Geometry check sheet. Reference: the model listing, model coordinates, mm. Face numbers are marked on the shaded views. A direction names the side the tool comes from. Give positions to 0.01 mm unless a question says otherwise; leave off trailing zeros. Loops run counter-clockwise (first coordinate to the right, second up) from the corner with the lowest first, then second, coordinate; pieces in that order, holes last. Notation, with made-up numbers: (87.5, 85.5) - (107.5, 85.5) arc R20 cw to (107.5, 122.5) - close; hole circle Ø4 at (59.25, 72.25). An arc over 180 degrees is marked (long way). One line per question, with ' | ' between items. Start each with the question number.
from build123d import *

# Parameters (mm, degrees)
F0_R     = 5
F1_DEPTH = 5
F2_W     = 3
F2_H     = 1.5
F3_DEPTH = 3
F4_R     = 0.5
F5_DEPTH = 25


with BuildPart() as f1:
    # F0 (on Top) → F1 (new body)
    with BuildSketch(Plane.XY):
        Circle(F0_R)
    extrude(amount=F1_DEPTH)

    # F2 (on face) → F3 (join)
    with BuildSketch(Plane.XY.offset(5)):
        with Locations((0, -2.75)):
            Rectangle(F2_W, F2_H)
    extrude(amount=F3_DEPTH)

    # F4 (on face) → F5 (cut)
    with BuildSketch(Plane.XY.offset(5)):
        Circle(F4_R)
    extrude(amount=-F5_DEPTH, mode=Mode.SUBTRACT)


solid = f1.part
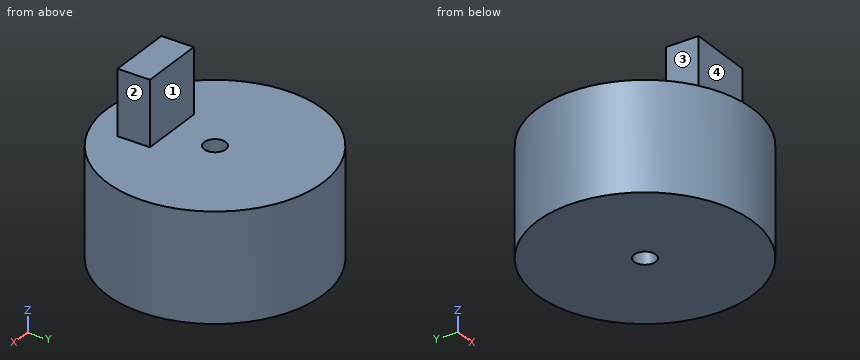
(1) Section check B-B, the plane z = 1. Record the boundary of the cut face in (x, y), and give its area (3 significant figures).
(2) Section check D-D, the plane x = 4. Record the boundary of the cut face in (y, z), and give its area (3 significant figures).
(3) Tool access check on the marked faces 1, 2, 3 and 4. Record the directions out of +Z, -Z, +X, -X, +Y, -Y that give a thin tool (end or side, any length) a straight path to the whole face; none if there is none.
(4) Depth check by flat-ended pin: pin 1 Ø1.6 at (y, z) = (-2.5, 6.5) entering from +X; pin 2 Ø5 at (x, y) = (2, 0.5) entering from +Z; pin 3 Ø1.6 at (y, z) = (-3, 7) entering from -X; pin 4 Ø6 at (x, y) = (2, 3) entering from -Z. Enter the tip coordinate at first touch or a pass-through.
(5) Material ranges on line 1 (Y direction, x = 0, z = 3.8); line 2 (Z direction, x = -1.75, y = -1.5); line 3 (X direction, y = -2.5, z = 6.5), recorded low to high.
(6) Section check C-C, the plane z = 5.25. Record the boundary of the cut face in (x, y).
(7) Section check A-A, the plane x = 0. Record the boundary of the cut face in (y, z).
Numbers:
1) outline: circle Ø10 at (0, 0); hole circle Ø1 at (0, 0) | area: 77.8 mm^2
2) outline: (-3, 0) - (3, 0) - (3, 5) - (-3, 5) - close | area: 30.0 mm^2
3) face 1: +Z, +X, -X, +Y | face 2: +Z, +X, +Y, -Y | face 3: +Z, -X, +Y, -Y | face 4: +Z, +X, -X, -Y
4) pin 1: x = 1.5 | pin 2: z = 5 | pin 3: x = -1.5 | pin 4: z = 0
5) line 1: -5 to -0.5, 0.5 to 5 | line 2: 0 to 5 | line 3: -1.5 to 1.5
6) outline: (-1.5, -3.5) - (1.5, -3.5) - (1.5, -2) - (-1.5, -2) - close
7) outline: (-5, 0) - (-0.5, 0) - (-0.5, 5) - (-2, 5) - (-2, 8) - (-3.5, 8) - (-3.5, 5) - (-5, 5) - close; (0.5, 0) - (5, 0) - (5, 5) - (0.5, 5) - close
